Study the drawing (mm; zero at the part's minimum x, y, z) and answer. A direction names the side the tool comes from. Give positions to 0.01 mm unless a question says otherwise; leave off trailing zeros. Order: outer loops, then holes, each group sorted by start corner. A loop starts at its lowest first (then second) coordinate and runs counter-clockwise, first axis right, second up. Notation, with made-up numbers: (-17, 7.5) - (37, 7.5) arc R32 ccw to (37, 36.5) - close; hole circle Ø10 at (-35.75, 16.25). An arc over 180 degrees is marked (long way). Put each result on its own line as item: value.
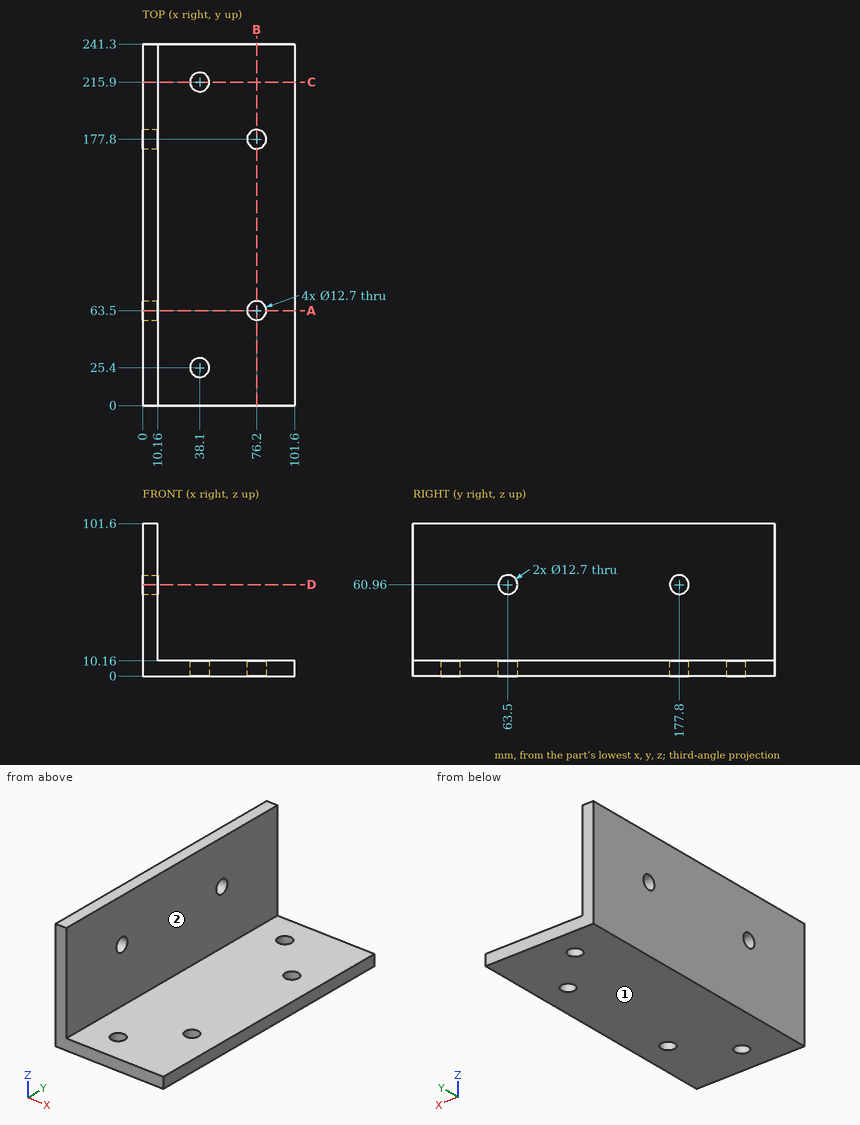
(1) Section A-A, the plane y = 63.5 is taken. Write down the section's boundary in (x, z), then the cut area to 3 significant figures.
Geometry check:
outline: (0, 0) - (69.85, 0) - (69.85, 10.16) - (10.16, 10.16) - (10.16, 54.61) - (0, 54.61) - close; (0, 67.31) - (10.16, 67.31) - (10.16, 101.6) - (0, 101.6) - close; (82.55, 0) - (101.6, 0) - (101.6, 10.16) - (82.55, 10.16) - close
area: 1,700 mm²
(2) A tool of negligible diameter and unlimited length cuts with its end or side. For the marked faces 1 and 2, from which of +Z, -Z, +X, -X, +Y, -Y can it reach the whole face along a straight path? Write none if from no direction.
Geometry check:
face 1: -Z, +X, -X, +Y, -Y
face 2: +Z, +X, +Y, -Y
(3) Section D-D, the plane z = 60.96 is taken. Write down the section's boundary in (x, y).
Geometry check:
outline: (0, 0) - (10.16, 0) - (10.16, 57.15) - (0, 57.15) - close; (0, 69.85) - (10.16, 69.85) - (10.16, 171.45) - (0, 171.45) - close; (0, 184.15) - (10.16, 184.15) - (10.16, 241.3) - (0, 241.3) - close
(4) Straight lines are drawn through the part: line 1 (Y direction, x = 38.1, z = 7.5); line 2 (Y direction, x = 6, z = 60); line 3 (X direction, y = 63, z = 8). For each, find the intervals that lie inside material, in ascending order.
Geometry check:
line 1: y = 0 to 19.05, 31.75 to 209.55, 222.25 to 241.3
line 2: y = 0 to 57.22, 69.78 to 171.52, 184.08 to 241.3
line 3: x = 0 to 69.87, 82.53 to 101.6
(5) Section B-B, the plane x = 76.2 is taken. Write down the section's boundary in (y, z).
Geometry check:
outline: (0, 0) - (57.15, 0) - (57.15, 10.16) - (0, 10.16) - close; (69.85, 0) - (171.45, 0) - (171.45, 10.16) - (69.85, 10.16) - close; (184.15, 0) - (241.3, 0) - (241.3, 10.16) - (184.15, 10.16) - close
(6) Section C-C, the plane y = 215.9 is taken. Write down the section's boundary in (x, z), then the cut area to 3 significant figures.
Geometry check:
outline: (0, 0) - (31.75, 0) - (31.75, 10.16) - (10.16, 10.16) - (10.16, 101.6) - (0, 101.6) - close; (44.45, 0) - (101.6, 0) - (101.6, 10.16) - (44.45, 10.16) - close
area: 1,830 mm²
(7) Given pin 1 (20.5 mm diameter, centred on x = 38.1, y = 215.9, fed in from -Z); pin 2 (3 mm diameter, centred on y = 62.5, z = 32.5, fed in from +X), each flat-ended and moving along its own axis, determine where each tip first touches the part or whether it passes through.
Geometry check:
pin 1: stops at z = 0
pin 2: stops at x = 10.16
